Could you check a few things on this model? Use its own coordinates, in mm. Face numbers are marked on the shaded views. A direction names the side the tool comes from. Give positions to 0.01 mm unless a question says otherwise; leave off trailing zeros. Loops run counter-clockwise (first coordinate to the right, second up) from the corner with the lowest first, then second, coordinate; pieces in that order, holes last. Notation, with made-up numbers: (15, -37.5) - (68, -37.5) arc R21 ccw to (68, -15.5) - close; hole circle Ø3 at (-4.75, -11.5). An arc over 180 degrees is marked (long way). One line per item, written item: value. Start each with the question number.
Q1. If I drill on line 1 (Y direction, x = -26, z = 7.65); line 2 (X direction, y = -6, z = 3.75); line 3 (X direction, y = -11.5, z = 16.5), over which ranges is the centre line in solid material (lowest first)? Write a range as from..to.
Q2. I want a section at A-A (y = 0). Please give me the cut outline in (x, z).
Q3. For the marked faces 1, 2, 3, 4 and 5, which set-ups out of +Z, -Z, +X, -X, +Y, -Y let a thin tool reach every point of the face, with its end or its side?
Q4. I want a section at B-B (x = -26). Please give me the cut outline in (y, z).
Q5. I'm going to push flat-ended pins straight in: P1, Ø6, axis at y = -4, z = 14, coming from the -X side; P2, Ø6, axis at x = 18, z = 16, coming from the +Y side; P3, Ø2, axis at x = -4.5, y = 3, coming from the +Z side; P4, Ø3, axis at x = 20.5, y = -10, coming from the +Z side. Where does each tip first touch, or does it pass through?
Q6. If we mould it in two halves opening along X, with no side actions, what happens to the marked faces 6, 7 and 8? For each: released by +X, released by -X, zero draft, split by the parting line, or undercut.
```python
from build123d import *

# Parameters (mm, degrees)
SKETCH1_R                                     = 14
EXTRUDE1_DEPTH                                = 10
SKETCH3_R                                     = 18.5
SKETCH3_R_2                                   = 14
EXTRUDE2_DEPTH                                = 15
EXTRUDE3_DEPTH                                = 7
CBORE_FOR_M3_PAN_HEAD_MACHINE_SCREW1_AT_COUNT = 2
CBORE_FOR_M3_PAN_HEAD_MACHINE_SCREW1_AT_PITCH = 14.99999999999997
EXTRUDE4_START                                = 20
SKETCH6_R                                     = 3.7499999999999996
EXTRUDE4_DEPTH                                = 20
FILLET1_R                                     = 2
SKETCH8_W                                     = 18.574175621006713
SKETCH8_H                                     = 7.448846743952753
EXTRUDE5_DEPTH                                = 15
FILLET2_R                                     = 3
EXTRUDE8_DEPTH                                = 5
F_2_9_2_9_DIAMETER_HOLE1_D                    = 2.9
F_2_9_2_9_DIAMETER_HOLE1_DEPTH                = 10
SKETCH14_W                                    = 6.5
SKETCH14_H                                    = 44.553858890679976
EXTRUDE9_DEPTH                                = 2
SKETCH15_R                                    = 1.45
EXTRUDE10_DEPTH                               = 10
SKETCH16_R                                    = 1.45
EXTRUDE11_DEPTH                               = 6


with BuildPart() as part:
    # Sketch1 → Extrude1 (new body)
    with BuildSketch(Plane.XY):
        with BuildLine():
            Line((-30, 21), (-22.199999999999996, 21))
            Line((-22.199999999999996, 21), (-22.199999999999996, 13.000000000000002))
            add(Edge.make_bspline(
                [(-22.199999999999996, 13.000000000000002), (-17.087298132677002, 13.293403264574941), (-3.0476406189760237, 14.099098854681937), (10.587905202926116, 17.638075889977564), (19.257911052248826, 19.88829395952834)],
                knots=[0, 0, 0, 0, 0.36416143786510685, 1, 1, 1, 1], degree=3))
            ThreePointArc((19.257911052248826, 19.88829395952834), (28.628449534780575, 20.83485668400702), (37.47030029247324, 17.590685353347904))
            add(Edge.make_bspline(
                [(44.90000000000001, 15), (43.95984253847409, 15.041510539741976), (41.267922149986155, 15.160366234496765), (38.96737663845901, 16.632619120705193), (37.47030029247324, 17.590685353347904)],
                knots=[0, 0, 0, 0, 0.3492515846852426, 1, 1, 1, 1], degree=3))
            Line((44.90000000000001, 15), (44.90000000000001, -15))
            add(Edge.make_bspline(
                [(44.90000000000001, -15), (43.95984253847409, -15.041510539741976), (41.267922149986155, -15.160366234496761), (38.96737663845901, -16.632619120705193), (37.47030029247324, -17.590685353347904)],
                knots=[0, 0, 0, 0, 0.3492515846852426, 1, 1, 1, 1], degree=3))
            ThreePointArc((37.47030029247324, -17.590685353347904), (28.628449534780575, -20.834856684007015), (19.257911052248826, -19.88829395952834))
            add(Edge.make_bspline(
                [(-22.199999999999996, -13.000000000000002), (-17.087298132677002, -13.293403264574941), (-3.0476406189760232, -14.099098854681936), (10.587905202926116, -17.638075889977564), (19.257911052248826, -19.88829395952834)],
                knots=[0, 0, 0, 0, 0.36416143786510685, 1, 1, 1, 1], degree=3))
            Line((-22.199999999999996, -13.000000000000002), (-22.199999999999996, -21))
            Line((-22.199999999999996, -21), (-30, -21))
            Line((-30, -21), (-30, 21))
        make_face()
        with Locations((26.000000000000004, 0)):
            Circle(SKETCH1_R, mode=Mode.SUBTRACT)
    extrude(amount=EXTRUDE1_DEPTH)

    # Sketch3 → Extrude2 (add)
    with BuildSketch(Plane.XY.offset(10)):
        with Locations(Location((26.000000000000004, 0, 0), (0, 0, 180))):
            Circle(SKETCH3_R)
        with Locations((26.000000000000004, 0)):
            Circle(SKETCH3_R_2, mode=Mode.SUBTRACT)
    extrude(amount=EXTRUDE2_DEPTH)

    # Sketch4 → Extrude3 (cut)
    with BuildSketch(Plane(origin=(0, 0, 0), x_dir=(-1, 0, 0), z_dir=(0, 0, -1))):
        Polygon((30, 23.412577815179247), (22, 23.412577815179247), (22.000000000000007, -25.98666339363831), (30.000000000000007, -25.98666339363831), align=None)
    extrude(amount=-EXTRUDE3_DEPTH, mode=Mode.SUBTRACT)

    # Sketch5 → CBORE for M3 Pan Head Machine Screw1 (revolve, cut)
    with BuildSketch(Plane(origin=(6.399999999999998, 7.499999999999986, 10), x_dir=(0, -1, 0), z_dir=(1, 0, 0))):
        Polygon((0, 0), (-2.45e-15, 9.999999999999998), (1.7999999999999978, 10), (1.7999999999999994, 4.999999999999999), (3.749999999999999, 4.999999999999999), (3.75, 0), align=None)
    cbore_for_m3_pan_head_machine_screw1 = revolve(axis=Axis((6.399999999999998, 7.499999999999986, 16.34999999999999), (0, 0, -1)), mode=Mode.SUBTRACT)

    # CBORE for M3 Pan Head Machine Screw1 at: CBORE for M3 Pan Head Machine Screw1 ×2
    with Locations(*[(0, -i * CBORE_FOR_M3_PAN_HEAD_MACHINE_SCREW1_AT_PITCH, 0) for i in range(1, CBORE_FOR_M3_PAN_HEAD_MACHINE_SCREW1_AT_COUNT)]):
        add(cbore_for_m3_pan_head_machine_screw1, mode=Mode.SUBTRACT)

    # Sketch6 → Extrude4 (cut)
    with BuildSketch(Plane.XY.offset(10).offset(EXTRUDE4_START)):
        with Locations((6.399999999999998, 7.499999999999986)):
            Circle(SKETCH6_R)
        with Locations((6.399999999999998, -7.499999999999984)):
            Circle(SKETCH6_R)
    extrude(amount=-EXTRUDE4_DEPTH, mode=Mode.SUBTRACT)

    # Fillet1
    fillet1_edges = [part.edges().sort_by_distance(p)[0] for p in [
        (7.957487706286119, -4.088734539094374, 17.5),
        (9.836860741750934, -9.000162738442441, 17.5),
        (9.836860741750938, 9.000162738442443, 17.5),
        (7.957487706286121, 4.088734539094375, 17.5),
    ]]
    fillet(fillet1_edges, radius=FILLET1_R)

    # Sketch8 → Extrude5 (cut)
    with BuildSketch(Plane.XY.offset(25)):
        with Locations((26, 19.72442337197638)):
            Rectangle(SKETCH8_W, SKETCH8_H)
        with Locations((26, -19.72442337197638)):
            Rectangle(SKETCH8_W, SKETCH8_H)
    extrude(amount=-EXTRUDE5_DEPTH, mode=Mode.SUBTRACT)

    # Fillet2
    fillet2_edges = [part.edges().sort_by_distance(p)[0] for p in [
        (35.28708781050336, 16, 17.5),
        (16.712912189496645, 16, 17.5),
        (35.28708781050336, -16, 17.5),
        (16.712912189496645, -16, 17.5),
    ]]
    fillet(fillet2_edges, radius=FILLET2_R)

    # Sketch11 → Extrude8 (cut)
    with BuildSketch(Plane.XY.offset(10)):
        with BuildLine():
            Line((26.000000000000004, 16.000000000000004), (26.000000000000004, 18.999999999999996))
            ThreePointArc((26.000000000000004, 18.999999999999996), (36.206280080860964, 16.025974132982387), (43.21742953366855, 8.034931253791655))
            Line((43.21742953366855, 8.034931253791655), (40.49888802835247, 6.766257897929818))
            ThreePointArc((40.49888802835247, 6.766257897929818), (34.5947621733566, 13.495557164616752), (26.000000000000004, 16.000000000000004))
        make_face()
        with BuildLine():
            Line((26.000000000000004, -16.000000000000004), (26.000000000000004, -18.999999999999996))
            ThreePointArc((26.000000000000004, -18.999999999999996), (15.793719919139045, -16.025974132982395), (8.782570466331453, -8.034931253791656))
            Line((8.782570466331453, -8.034931253791656), (11.501111971647536, -6.766257897929817))
            ThreePointArc((11.501111971647536, -6.766257897929817), (17.405237826643408, -13.495557164616757), (26.000000000000004, -16.000000000000004))
        make_face()
    extrude(amount=EXTRUDE8_DEPTH, mode=Mode.SUBTRACT)

    # Ø2.9 (2.9) Diameter Hole1
    with Locations(Plane(origin=(-26, -17.85, 10), x_dir=(1, 0, 0), z_dir=(0, 0, 1))):
        with Locations((0, 0), (0, 10.35), (0, 25.35), (0, 35.7)):
            Hole(F_2_9_2_9_DIAMETER_HOLE1_D / 2, depth=F_2_9_2_9_DIAMETER_HOLE1_DEPTH)

    # Sketch14 → Extrude9 (cut)
    with BuildSketch(Plane.XY.offset(10)):
        with Locations((-6.350000000000001, -1.057050154528838)):
            Rectangle(SKETCH14_W, SKETCH14_H)
    extrude(amount=-EXTRUDE9_DEPTH, mode=Mode.SUBTRACT)

    # Sketch15 → Extrude10 (cut)
    with BuildSketch(Plane.XY.offset(8)):
        with Locations((-6.500000000000001, 1.73e-15)):
            Circle(SKETCH15_R)
    extrude(amount=-EXTRUDE10_DEPTH, mode=Mode.SUBTRACT)

    # Sketch16 → Extrude11 (cut)
    with BuildSketch(Plane(origin=(44.90000000000001, 0, 0), x_dir=(0, 0, -1), z_dir=(1, 0, 0))):
        with Locations((-5, -11)):
            Circle(SKETCH16_R)
        with Locations((-5, 11)):
            Circle(SKETCH16_R)
    extrude(amount=-EXTRUDE11_DEPTH, mode=Mode.SUBTRACT)


solid = part.part
```
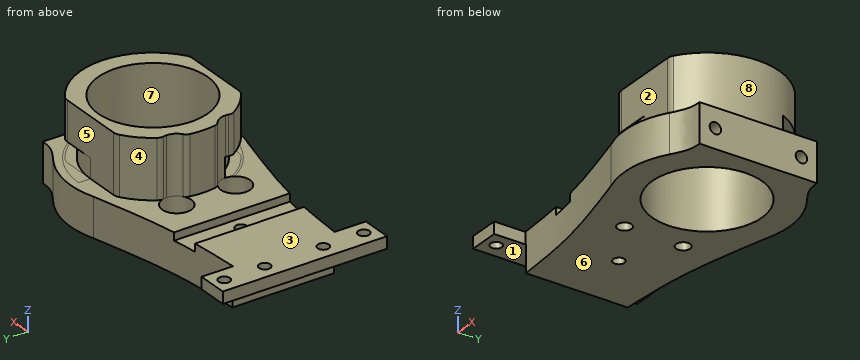
Worked answers:
1. line 1: y = -21..-19.3, -16.4..-8.95, -6.05..6.05, 8.95..16.4, 19.3..21
1. line 2: x = -22..5.41, 7.39..13.35, 38.65..44.9
1. line 3: x = 11.51..18.02, 33.98..40.49
2. outline: (-30, 7) - (-22, 7) - (-22, 0) - (-7.95, 0) - (-7.95, 8) - (-9.6, 8) - (-9.6, 10) - (-30, 10) - close; (-5.05, 0) - (12, 0) - (12, 25) - (7.5, 25) - (7.5, 10) - (-3.1, 10) - (-3.1, 8) - (-5.05, 8) - close; (40, 0) - (44.9, 0) - (44.9, 10) - (44.5, 10) - (44.5, 25) - (40, 25) - close
3. face 1: -Z, -X, +Y, -Y
3. face 2: +Z, +X, -X, -Y
3. face 3: +Z, -X, +Y, -Y
3. face 4: +Z, -X, +Y
3. face 5: +Z, +X, -X, +Y
4. outline: (-21, 7) - (-19.3, 7) - (-19.3, 10) - (-21, 10) - close; (-16.4, 7) - (-8.95, 7) - (-8.95, 10) - (-16.4, 10) - close; (-6.05, 7) - (6.05, 7) - (6.05, 10) - (-6.05, 10) - close; (8.95, 7) - (16.4, 7) - (16.4, 10) - (8.95, 10) - close; (19.3, 7) - (21, 7) - (21, 10) - (19.3, 10) - close
5. P1: stops at x = 7.53
5. P2: stops at y = 16
5. P3: stops at z = 8
5. P4: passes through
6. face 6: zero draft
6. face 7: undercut
6. face 8: released by +X
